```python
from build123d import *

# Parameters (mm, degrees)
F1_DEPTH       = 60
F3_D           = 4.5
F3_CBORE_D     = 7.6
F3_CBORE_DEPTH = 4.3
F4_R           = 0.5


with BuildPart() as f1:
    # F0 (on Front) → F1 (new body)
    with BuildSketch(Plane.XZ):
        Polygon((0, -5.126866), (0, 17.873134), (-1.5, 17.873134), (-1.5, 32.873134), (-3.5, 32.873134), (-3.5, 2.873134), (-12.5, 2.873134), (-12.5, -5.126866), align=None)
        Polygon((1.5, 17.873134), (0, 17.873134), (0, -5.126866), (12.5, -5.126866), (12.5, 2.873134), (3.5, 2.873134), (3.5, 32.873134), (1.5, 32.873134), align=None)
    extrude(amount=F1_DEPTH)

    # F3 (through all)
    with Locations(Plane.XY.offset(2.873134)):
        with Locations((-8, -50), (-8, -10), (8, -50), (8, -10)):
            CounterBoreHole(F3_D / 2, F3_CBORE_D / 2, F3_CBORE_DEPTH)

    # F4
    f4_edges = [f1.edges().sort_by_distance(p)[0] for p in [
        (-1.5, -60, 25.373134),
        (1.5, -60, 25.373134),
        (2.5, -60, 32.873134),
        (-2.5, -60, 32.873134),
    ]]
    fillet(f4_edges, radius=F4_R)


solid = f1.part
```
Can you work these out from the model? Positions are in its coordinate system, mm. A direction names the side the tool comes from. Give positions to 0.01 mm unless a question says otherwise; leave off trailing zeros. Write each loop counter-clockwise with the first axis right and the second up, starting at its lowest first coordinate (ties: lowest second). Pieces come first, ordered by that corner, then holes. Notation, with made-up numbers: (-33.5, 88.5) -> (18.5, 88.5) arc R26 cw to (18.5, 121.5) -> close; hole circle Ø3 at (84, 41). An arc over 180 degrees is marked (long way). Write item = value, one per line.
(1) For faces 1 (the face through (8, -30, 2.873)), 2 (the face through (7.51, -6.23, 0.75)), 3 (the face through (-1.5, -29, 25)), which set-ups out of +Z, -Z, +X, -X, +Y, -Y let a thin tool reach every point of the face, with its end or its side?
Worked out:
face_1 = +Z, +X, +Y, -Y
face_2 = +Z
face_3 = +Z, +Y, -Y
(2) Thinking about a two-plate mould opening in X: for faces 4 (the face through (-8, -30, 2.873)), 5 (the face through (-3.5, -30, 18)), 6 (the face through (1.5, -29, 25)), 7 (the face through (10, -12, -1.427)), which applies, released by +X, released by -X, zero draft, split by the parting line, or undercut?
Worked out:
face_4 = zero draft
face_5 = released by -X
face_6 = undercut
face_7 = undercut
(3) Suppose I cut it at D-D on y = -28.5. Write out the boundary of the cut face in (x, z), then the cut area to 3 significant figures.
Worked out:
outline = (-12.5, -5.13) -> (12.5, -5.13) -> (12.5, 2.87) -> (3.5, 2.87) -> (3.5, 32.87) -> (1.5, 32.87) -> (1.5, 17.87) -> (-1.5, 17.87) -> (-1.5, 32.87) -> (-3.5, 32.87) -> (-3.5, 2.87) -> (-12.5, 2.87) -> close
area = 365 mm^2
(4) I'm going to push flat-ended pins straight in: P1, Ø4, axis at x = -8.5, y = -48.5, coming from the +Z side; P2, Ø1.5, axis at y = -34.5, z = 6, coming from the -X side; P3, Ø15, axis at y = -21.5, z = 22.5, coming from the +X side. Where does each tip first touch, or does it pass through?
Worked out:
P1 = -1.43
P2 = -3.5
P3 = 3.5
(5) I need wall thicknesses on probe 1 along Y at (x, z) = (-8, -2.6); probe 2 along Y at (x, z) = (8, 1.2); probe 3 along X at (y, z) = (-42, 6). Which ranges of each line are inside material? Lowest first, please. Write a range as from..to.
Worked out:
probe_1 = -60..-52.25, -47.75..-12.25, -7.75..0
probe_2 = -60..-53.8, -46.2..-13.8, -6.2..0
probe_3 = -3.5..3.5
(6) Suppose I cut it at A-A on x = -8. Write out the boundary of the cut face in (y, z).
Worked out:
outline = (-60, -5.13) -> (-52.25, -5.13) -> (-52.25, -1.43) -> (-53.8, -1.43) -> (-53.8, 2.87) -> (-60, 2.87) -> close; (-47.75, -5.13) -> (-12.25, -5.13) -> (-12.25, -1.43) -> (-13.8, -1.43) -> (-13.8, 2.87) -> (-46.2, 2.87) -> (-46.2, -1.43) -> (-47.75, -1.43) -> close; (-7.75, -5.13) -> (0, -5.13) -> (0, 2.87) -> (-6.2, 2.87) -> (-6.2, -1.43) -> (-7.75, -1.43) -> close
(7) Suppose I cut it at C-C on z = 20. Write out the boundary of the cut face in (x, y).
Worked out:
outline = (-3.5, -60) -> (-2, -60) arc R0.5 ccw to (-1.5, -59.5) -> (-1.5, 0) -> (-3.5, 0) -> close; (1.5, -59.5) arc R0.5 ccw to (2, -60) -> (3.5, -60) -> (3.5, 0) -> (1.5, 0) -> close
(8) Suppose I cut it at B-B on y = -50. Write out the boundary of the cut face in (x, z).
Worked out:
outline = (-12.5, -5.13) -> (-10.25, -5.13) -> (-10.25, -1.43) -> (-11.8, -1.43) -> (-11.8, 2.87) -> (-12.5, 2.87) -> close; (-5.75, -5.13) -> (5.75, -5.13) -> (5.75, -1.43) -> (4.2, -1.43) -> (4.2, 2.87) -> (3.5, 2.87) -> (3.5, 32.87) -> (1.5, 32.87) -> (1.5, 17.87) -> (-1.5, 17.87) -> (-1.5, 32.87) -> (-3.5, 32.87) -> (-3.5, 2.87) -> (-4.2, 2.87) -> (-4.2, -1.43) -> (-5.75, -1.43) -> close; (10.25, -5.13) -> (12.5, -5.13) -> (12.5, 2.87) -> (11.8, 2.87) -> (11.8, -1.43) -> (10.25, -1.43) -> close
